Work out the finished part from the listing and answer in its coordinate system (mm). A direction names the side the tool comes from. Give positions to 0.01 mm unless a question says otherwise; leave off trailing zeros. Write each loop counter-clockwise with the first axis right and the second up, starting at its lowest first coordinate (ties: lowest second). Pieces come first, ordered by that corner, then holes. Notation, with made-up numbers: (66.25, -15) -> (91.25, -15) arc R16 ccw to (91.25, -9) -> close; hole circle Ø11 at (55.5, -28). An arc over 180 degrees is marked (long way). Write item = value, one per line. Start each with the question number.
from build123d import *

# Parameters (mm, degrees)
M4X0_7_TAPPED_HOLE1_D = 3.3


with BuildPart() as part:
    # Sketch2 → Revolve1 (revolve)
    with BuildSketch(Plane.XY):
        Polygon((0, 37.6), (41.5, 37.6), (41.5, 20), (44, 20), (44, 18), (48, 18), (48, 42.5), (22, 42.5), (22, 45), (5, 45), (5, 55), (0, 55), (0, 45), align=None)
    revolve(axis=Axis((-64.103352454, 0, 0), (1, 0, 0)))

    # M4x0.7 Tapped Hole1 (through all)
    with Locations(Plane.ZY):
        with Locations((0, 50), (50, 0), (0, -50), (-50, 0)):
            Hole(M4X0_7_TAPPED_HOLE1_D / 2)


solid = part.part
(1) For faces 4 (the cylindrical face through (34.818, -33.727, -25.861)), 5 (the cylindrical face through (21.04, -8.151, -36.706)), 6 (the cylindrical face through (2.53, 51.39, -0.89)), determine the directions among +Z, -Z, +X, -X, +Y, -Y from which every point of the face is accessible in a straight line to the end or side of a thin tool.
(2) A cutting plane is placed at A-A, the plane y = 0. State how many separate pieces and enclosed holes the cut face has, then the cut area to 3 significant figures.
(3) Determine the mould class of faces 1 (the cylindrical face through (2.53, 0.07, -48.35)), 2 (the flat face through (22, 26.9, -33.1)), 3 (the cylindrical face through (13.381, 20.765, -39.923)) for opening direction Y: pulls with the +Y half, pulls with the -Y half, needs draft (parallel to the pull), parting line crosses it, or undercut.
(4) A cutting plane is placed at C-C, the plane y = 50. Write down the section's boundary in (x, z).
(5) Each of these flat-tipped pins is pushed along its axis until it touches: pin 1 (1 mm diameter, centred on y = -16, z = 16.5, fed in from -X); pin 2 (21.5 mm diameter, centred on y = 0, z = 0, fed in from +X); pin 3 (1.5 mm diameter, centred on x = 19.5, y = -38.5, fed in from -Z); pin 4 (5.5 mm diameter, centred on y = 0, z = -50, fed in from +X). Where does it stop, or does it pass through?
(6) Find the intervals of material crossed by line 1 along Z through (x, y) = (46.5, 0); line 2 along Z through (x, y) = (42, 0); line 3 along X through (y, z) = (22, 16), in increasing order.
Results list:
q1.face_4 = +X
q1.face_5 = -X
q1.face_6 = +X, -X
q2.separate_pieces = 4
q2.enclosed_holes = 0
q2.area = 892 mm²
q3.face_1 = undercut
q3.face_2 = needs draft
q3.face_3 = parting line crosses it
q4.outline = (0, -22.91) -> (5, -22.91) -> (5, -1.65) -> (0, -1.65) -> close; (0, 1.65) -> (5, 1.65) -> (5, 22.91) -> (0, 22.91) -> close
q5.pin_1 = 41.5
q5.pin_2 = through
q5.pin_3 = -24.49
q5.pin_4 = 5
q6.line_1 = -42.5 to -18, 18 to 42.5
q6.line_2 = -42.5 to -20, 20 to 42.5
q6.line_3 = 41.5 to 48
